For this review, take the finished solid that the model builds, in its own axes (mm). Face numbers are marked on the shaded views. A direction names the side the tool comes from. Round coordinates to 2 decimals unless told otherwise and drop trailing zeros. Order: outer loops, then holes, each group sorted by start corner. A loop starts at its lowest first (then second) coordinate and runs counter-clockwise, first axis right, second up. Notation, with made-up numbers: (47, -5) - (92, -5) arc R16 cw to (92, 1) - close; hole circle Ø11 at (-14, 54). An arc over 180 degrees is marked (long way). Write each question's results on one line, items separated by ' | '. Start each with the question number.
(1) For the marked faces 5 and 6, list the 3-axis set-ups (+Z, -Z, +X, -X, +Y, -Y) from which the entire face can be reached by the end or side of a thin tool; tool diameter is ignored.
(2) Take a section at A-A, the plane y = 347. Give the boundary of the cut face in (x, z), plus the area to 3 significant figures.
(3) Draft analysis for pull direction Z (two halves, no side actions). For the marked faces 1, 2, 3 and 4, state which applies: pulls with the +Z half, pulls with the -Z half, needs draft (parallel to the pull), parting line crosses it, or undercut.
(4) Take a section at B-B, the plane x = -181.5. Give the boundary of the cut face in (y, z), plus the area to 3 significant figures.
(5) Take a section at D-D, the plane y = -41. Give the boundary of the cut face in (x, z), plus the area to 4 significant figures.
(6) Insertion check: pin 1 Ø13 at (y, z) = (85.5, 301) entering from +X; pin 2 Ø10 at (x, z) = (-91.5, 312) entering from -Y; pin 3 Ø17.5 at (y, z) = (84, 314) entering from -X. Each pin has a flat end and moves straight along its axis. Give the tip position at first contact, or say it passes through.
(7) Take a section at C-C, the plane z = -272.5. Give the boundary of the cut face in (x, y).
(8) For L1, parallel to X at y = 376.5, z = -267.5; L2, parallel to Y at x = -132, z = -266.5; L3, parallel to Y at x = 84.5, z = -212.5, list the stretches that pass through material, from the lowest coordinate up. Write a range as from..to.
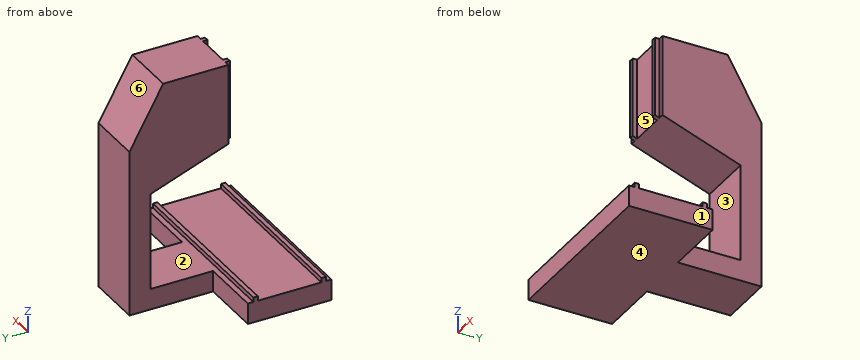
Autodesk Inventor part; units mm, degrees
ref_plane "YZ Plane" through (0, 0, 0) normal (1, 0, 0) x (0, 1, 0)
ref_plane "XZ Plane" through (0, 0, 0) normal (0, 1, 0) x (-1, 0, 0)
ref_plane "XY Plane" through (0, 0, 0) normal (0, 0, 1) x (1, 0, 0)
sketch "Sketch1" plane through (0, 0, 0) normal (1, 0, 0) x (0, 1, 0)
  line L0 (0, 9.8901) -> (0, -9.3874)
  line L1 (-150, -257) -> (150, -257)
  line L2 (150, -257) -> (150, -332)
  line L3 (150, -332) -> (-150, -332)
  line L4 (-150, -332) -> (-150, -257)
  point P0 (0, 0)
  dimension "d0" = 257
  dimension "d1" = 300
  dimension "d2" = 75
extrude "Extrusion1" add sketch "Sketch1" along normal mid plane 650
sketch "Sketch2" plane through (0, 0, 0) normal (1, 0, 0) x (0, 1, 0)
  line L0 (450, -332) -> (450, 268)
  line L1 (450, 268) -> (328.8182, 483)
  line L2 (295, 543) -> (95, 543) construction
  line L3 (95, 483) -> (95, 193)
  line L4 (95, 193) -> (375, 193) construction
  line L5 (375, 91.0981) -> (375, -257)
  line L6 (-150, -332) -> (150, -332)
  line L7 (150, -332) -> (150, -257)
  line L8 (150, -332) -> (450, -332)
  line L9 (150, -257) -> (-150, -257)
  line L10 (150, -332) -> (150, -257)
  line L11 (150, -257) -> (150, -332)
  line L12 (150, -257) -> (375, -257)
  line L13 (95, 193) -> (375, 91.0981)
  line L14 (328.8182, 483) -> (95, 483)
  point P0 (0, 0)
  dimension "d7" = 75
  dimension "d8" = 300
  dimension "d9" = 600
  dimension "d10" = 280
  dimension "d11" = 450
  dimension "d12" = 350
  dimension "d13" = 200
  dimension "d22" = 60
extrude "Extrusion2" add sketch "Sketch2" along normal mid plane 200
sketch "Sketch3" plane through (-325, 0, 0) normal (-1, 0, 0) x (0, 0, 1)
  line L0 (-257, 150) -> (-257, -150)
  line L1 (-241, 130) -> (-257, 130)
  line L2 (-257, 130) -> (-257, 114)
  line L3 (-257, 114) -> (-241, 114)
  line L4 (-241, 114) -> (-241, 130)
  line L5 (-257, 150) -> (-332, 150)
  line L6 (-111.2497, 0) -> (-314.6527, 0)
  line L7 (-241, -130) -> (-257, -130)
  line L8 (-257, -130) -> (-257, -114)
  line L9 (-257, -114) -> (-241, -114)
  line L10 (-241, -114) -> (-241, -130)
  point P0 (0, 0)
  dimension "d23" = 20
  dimension "d24" = 16
  dimension "d25" = 16
extrude "Extrusion3" add sketch "Sketch3" against normal up to surface (650 mm away)
sketch "Sketch4" plane through (-100, 95, 483) normal (0, 0, 1) x (1, 0, 0)
  line L0 (100, -95) -> (100, 134.7598)
  line L1 (0, 0) -> (200, 0)
  line L2 (20, 0) -> (36, 0)
  line L3 (36, 0) -> (36, -16)
  line L4 (36, -16) -> (20, -16)
  line L5 (20, -16) -> (20, 0)
  line L6 (0, 0) -> (0, 233.8182)
  line L7 (180, 0) -> (164, 0)
  line L8 (164, 0) -> (164, -16)
  line L9 (164, -16) -> (180, -16)
  line L10 (180, -16) -> (180, 0)
  point P0 (36, 0)
  dimension "d28" = 20
  dimension "d29" = 16
  dimension "d30" = 16
extrude "Extrusion4" add sketch "Sketch4" against normal up to surface surface through (0, 95, 193) normal (0, -0.342, -0.9397)
properties part number "base"
Results below:
1) face 5: +Z, -Y | face 6: +Z, +X, -X, +Y
2) outline: (-100, -332) - (100, -332) - (100, -257) - (-100, -257) - close; (-100, 101.29) - (100, 101.29) - (100, 450.74) - (-100, 450.74) - close | area: 84,900 mm^2
3) face 1: needs draft | face 2: undercut | face 3: undercut | face 4: pulls with the -Z half
4) outline: (-150, -332) - (150, -332) - (150, -257) - (130, -257) - (130, -241) - (114, -241) - (114, -257) - (-114, -257) - (-114, -241) - (-130, -241) - (-130, -257) - (-150, -257) - close | area: 23,000 mm^2
5) outline: (-325, -332) - (325, -332) - (325, -257) - (-325, -257) - close | area: 48,750 mm^2
6) pin 1: stops at x = 80 | pin 2: stops at y = 95 | pin 3: stops at x = -80
7) outline: (-325, -150) - (325, -150) - (325, 150) - (100, 150) - (100, 450) - (-100, 450) - (-100, 150) - (-325, 150) - close
8) L1: x = -100..100 | L2: y = -150..150 | L3: y = 375..450
